For this review, take the finished solid that the model builds, in its own axes (mm). Round coordinates to 2 decimals unless told otherwise and drop trailing zeros. Order: outer loops, then holes, each group sorted by start corner. A loop starts at its lowest first (then second) coordinate and runs counter-clockwise, first axis right, second up.
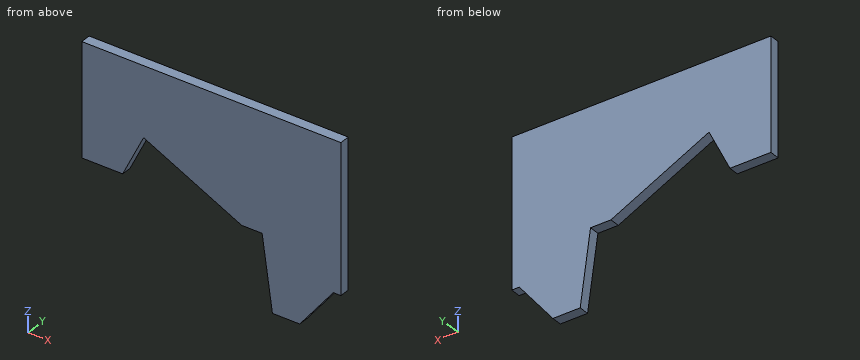
Autodesk Inventor part; units mm, degrees
ref_plane "YZ Plane" through (0, 0, 0) normal (1, 0, 0) x (0, 1, 0)
ref_plane "XZ Plane" through (0, 0, 0) normal (0, 1, 0) x (-1, 0, 0)
ref_plane "XY Plane" through (0, 0, 0) normal (0, 0, 1) x (1, 0, 0)
sketch "Sketch1" plane through (0, 0, 0) normal (0, 1, 0) x (-1, 0, 0)
  line L0 (0, 0) -> (482.6, 0)
  line L1 (482.6, 0) -> (482.6, -209.55)
  line L2 (482.6, -209.55) -> (406.4, -209.55)
  line L3 (406.4, -209.55) -> (367.4288, -129.6472)
  line L4 (367.4288, -129.6472) -> (184.7939, -218.7242)
  line L5 (184.7939, -218.7242) -> (146.6939, -218.7242)
  line L6 (146.6939, -218.7242) -> (127.4536, -355.6254)
  line L7 (127.4536, -355.6254) -> (76.6536, -355.6254)
  line L8 (76.6536, -355.6254) -> (14.1024, -275.5635)
  line L9 (14.1024, -275.5635) -> (0, -275.5635)
  line L10 (0, 0) -> (0, -275.5635)
  point P0 (438.8308, 0)
  point P1 (482.6, -106.5112)
  dimension "d22" = 98
  dimension "d23" = 154
  dimension "d26" = 76.2
  dimension "d27" = 128
  dimension "d29" = 355.6254
  dimension "d30" = 88.9
  dimension "d33" = 203.2
  dimension "d34" = 38.1
  dimension "d35" = 50.8
  dimension "d36" = 101.6
  dimension "d37" = 138.2466
  dimension "d38" = 209.55
  dimension "d39" = 482.6
extrude "Extrusion1" add sketch "Sketch1" along normal blind 19.05
properties part number "Side Panel"
Q1. Take a section at C-C, the plane x = -164. State the section outline as (y, z) points, plus the area to 3 significant figures.
Q2. Clearance check with flat-ended pins moving along their axes: pin 1 (4 mm diameter, centred on x = -9, y = 5, fed in from -Z); pin 2 (9.5 mm diameter, centred on x = -167.5, y = 7.5, fed in from -Z); pin 3 (5 mm diameter, centred on x = -337, y = 11, fed in from -Z). State where each tip first meets the part, or that it passes through.
Q3. Take a section at D-D, the plane z = -180.5. State the section outline as (x, y) points.
Q4. Wall thickness on line 1 (X direction, y = 5, z = -142.5); line 2 (X direction, y = 6, z = -165.5); line 3 (Z direction, x = -332.5, y = 15.25): over which ranges is each line inside the solid? List them lowest first.
Q5. Take a section at A-A, the plane z = -144.5. State the section outline as (x, y) points, plus the area to 3 significant figures.
Q6. Take a section at B-B, the plane y = 14.25. State the section outline as (x, z) points.
Working result:
1. outline: (0, -218.72) - (19.05, -218.72) - (19.05, 0) - (0, 0) - close
1. area: 4,170 mm2
2. pin 1: stops at z = -275.56
2. pin 2: stops at z = -218.72
2. pin 3: stops at z = -145.71
3. outline: (-482.6, 0) - (-392.23, 0) - (-392.23, 19.05) - (-482.6, 19.05) - close; (-263.17, 0) - (0, 0) - (0, 19.05) - (-263.17, 19.05) - close
4. line 1: x = -482.6 to -373.7, -341.08 to 0
4. line 2: x = -482.6 to -384.92, -293.92 to 0
4. line 3: z = -146.68 to 0
5. outline: (-482.6, 0) - (-374.67, 0) - (-374.67, 19.05) - (-482.6, 19.05) - close; (-336.98, 0) - (0, 0) - (0, 19.05) - (-336.98, 19.05) - close
5. area: 8,480 mm2
6. outline: (-482.6, -209.55) - (-406.4, -209.55) - (-367.43, -129.65) - (-184.79, -218.72) - (-146.69, -218.72) - (-127.45, -355.63) - (-76.65, -355.63) - (-14.1, -275.56) - (0, -275.56) - (0, 0) - (-482.6, 0) - close
